Geometry: final body of the model. Coordinates: model frame, mm. A direction names the side the tool comes from. Round coordinates to 2 decimals unless told otherwise and drop trailing zeros. Order: outer loops, then holes, each group sorted by start corner. A loop starts at its lowest first (then second) coordinate and runs counter-clockwise, first axis right, second up. Notation, with made-up numbers: (55, -6.5) - (72, -6.5) arc R11 ccw to (72, 13.5) - close; hole circle Ø9 at (2.25, 85). An arc over 180 degrees is marked (long way). Put each result on its own line as item: value. Start each with the question number.
(1) Section D-D (y = 10.25). Output: boundary loops of the cut face in (x, z), and give its area (3 significant figures).
(2) Pin query (flat end, axial travel): P1, Ø1.5, axis at x = -0.5, z = -7.5, coming from the +Y side; P2, Ø4, axis at y = 3, z = -6, coming from the -X side; P3, Ø10, axis at y = 9.5, z = -38.5, coming from the +X side. Return the tip coordinate at first contact, or that it passes through.
(3) Pull-direction query (X, two-part tool) for faces 1 (the face through (5, 0, 11)), 2 (the face through (2.028, -3.448, 8.288)), 3 (the face through (0, -6, -39)); classes: released by +X, released by -X, zero draft, split by the parting line, or undercut.
(4) Section A-A (y = 0). Output: boundary loops of the cut face in (x, z) (3 decimals).
(5) Access query for faces 4 (the face through (8, -3, 0)), 5 (the face through (0, 0, -48)), 6 (the face through (0, 0, 5.5)). Directions: +Z, -Z, +X, -X, +Y, -Y. A direction counts if a zero-diameter tool reaches every point of the face in a straight line with its end or side. Return the directions, or none.
(6) Material intervals for L1, parallel to X at y = 0.5, z = 7; L2, parallel to Z at x = -8.5, y = 6.5; L3, parallel to X at y = 6.25, z = -10, sorted ascending. Write a range as [from, to].
(7) Section C-C (x = 6.75). Output: boundary loops of the cut face in (y, z).
(8) Section B-B (z = -18.5). Output: boundary loops of the cut face in (x, y).
Solid Edge part; units mm, degrees
sketch "Sketch1" plane through (0, 0, 0) normal (0, 0, 1) x (1, 0, 0)
  circle A0 centre (0, 0) radius 12.165
extrude "Protrusion1" add sketch "Sketch1" along normal blind 11
sketch "Sketch2" plane through (0, 0, 11) normal (0, 0, 1) x (1, 0, 0)
  line L0 (0, -4.6188) -> (-4, -2.3094)
  line L1 (-4, -2.3094) -> (-4, 2.3094)
  line L2 (-4, 2.3094) -> (0, 4.6188)
  line L3 (0, 4.6188) -> (4, 2.3094)
  line L4 (4, 2.3094) -> (4, -2.3094)
  line L5 (4, -2.3094) -> (0, -4.6188)
extrude "Cutout1" cut sketch "Sketch2" against normal blind 5.5
sketch "Sketch3" plane through (0, 0, 0) normal (0, 0, -1) x (0, 1, 0)
  circle A0 centre (0, 0) radius 8
extrude "Protrusion2" add sketch "Sketch3" along normal blind 30
sketch "Sketch4" plane through (0, 0, -30) normal (0, 0, -1) x (0, 1, 0)
  circle A0 centre (0, 0) radius 6
extrude "Protrusion3" add sketch "Sketch4" along normal blind 18
chamfer "Chamfer1" distance 0.5 angle 45 1 edges at (0, -6, -48)
properties part number "108084"
Checks:
1. outline: (-6.55, 0) - (6.55, 0) - (6.55, 11) - (-6.55, 11) - close
1. area: 144 mm²
2. P1: stops at y = 8
2. P2: stops at x = -7.94
2. P3: stops at x = 3.97
3. face 1: zero draft
3. face 2: undercut
3. face 3: split by the parting line
4. outline: (-12.165, 0) - (-8, 0) - (-8, -30) - (-6, -30) - (-6, -47.5) - (-5.5, -48) - (5.5, -48) - (6, -47.5) - (6, -30) - (8, -30) - (8, 0) - (12.165, 0) - (12.165, 11) - (4, 11) - (4, 5.5) - (-4, 5.5) - (-4, 11) - (-12.165, 11) - close
5. face 4: -Z
5. face 5: -Z, +X, -X, +Y, -Y
5. face 6: +Z
6. L1: x = [-12.15, -4], [4, 12.15]
6. L2: z = [0, 11]
6. L3: x = [-4.99, 4.99]
7. outline: (-10.12, 0) - (-4.29, 0) - (-4.29, -30) - (4.29, -30) - (4.29, 0) - (10.12, 0) - (10.12, 11) - (-10.12, 11) - close
8. outline: circle Ø16 at (0, 0)
